Here's how the part is built. I have some questions about the finished solid (model axes, mm). A direction names the side the tool comes from. Coordinates: 2 decimals unless noted, no trailing zeros. Write each loop counter-clockwise with the first axis right and the second up, starting at its lowest first coordinate (ties: lowest second). Pieces come first, ordered by that corner, then holes.
Item 1: If we section it at D-D (z = 6.25): Please give me the cut outline in (x, y), then the cut area to 3 significant figures.
Item 2: We'd pull the mould along X, two halves only. Please class faces 3 (the face through (5, 2, 4)), 4 (the face through (-35, 2, 0)), 5 (the face through (35, 2, 0)), 6 (the face through (0, 2, 10)): +X half, -X half, draft (parallel to the pull), parting line (faces both ways), or undercut.
Item 3: If we section it at B-B (z = -3): Please give me the cut outline in (x, y), then the cut area to 3 significant figures.
Item 4: If we section it at A-A (x = -28.55): Please give me the cut outline in (y, z), then the cut area to 3 significant figures.
Item 5: For faces 1 (the face through (-5, 2, 4)), 2 (the face through (0, 2, -10)), which set-ups out of +Z, -Z, +X, -X, +Y, -Y let a thin tool reach every point of the face, with its end or its side?
Item 6: If we section it at C-C (y = 0.7): Please give me the cut outline in (x, z), then the cut area to 3 significant figures.
Item 7: If I drill on line 1 (X direction, y = 2, z = 1.5); line 2 (X direction, y = 3.05, z = -3); line 3 (Z direction, x = -30.5, y = 3.9), over which ranges is the centre line in solid material (lowest first)?
from build123d import *

# Parameters (mm, degrees)
SKETCH_1_W      = 70
SKETCH_1_H      = 20
SKETCH_1_R      = 3
SKETCH_1_W_2    = 2
SKETCH_1_H_2    = 7
EXTRUDE_1_DEPTH = 5


with BuildPart() as part:
    # 草图1 → 凸台-拉伸1 (new body)
    with BuildSketch(Plane(origin=(0, 0, 0), x_dir=(1, 0, 0), z_dir=(0, 1, 0))):
        Rectangle(SKETCH_1_W, SKETCH_1_H)
        with Locations(Location((-28.55, 3, 0), (0, 0, 270))):
            Circle(SKETCH_1_R, mode=Mode.SUBTRACT)
        with Locations(Location((28.55, 3, 0), (0, 0, 270))):
            Circle(SKETCH_1_R, mode=Mode.SUBTRACT)
        with Locations((-6, -3.5)):
            Rectangle(SKETCH_1_W_2, SKETCH_1_H_2, mode=Mode.SUBTRACT)
        with Locations((6, -3.5)):
            Rectangle(SKETCH_1_W_2, SKETCH_1_H_2, mode=Mode.SUBTRACT)
    extrude(amount=EXTRUDE_1_DEPTH)


solid = part.part
Answer list:
1. outline: (-35, 0) - (-7, 0) - (-7, 5) - (-35, 5) - close; (-5, 0) - (5, 0) - (5, 5) - (-5, 5) - close; (7, 0) - (35, 0) - (35, 5) - (7, 5) - close
1. area: 330 mm2
2. face 3: undercut
2. face 4: -X half
2. face 5: +X half
2. face 6: draft
3. outline: (-35, 0) - (-31.55, 0) - (-31.55, 5) - (-35, 5) - close; (-25.55, 0) - (25.55, 0) - (25.55, 5) - (-25.55, 5) - close; (31.55, 0) - (35, 0) - (35, 5) - (31.55, 5) - close
3. area: 290 mm2
4. outline: (0, -10) - (5, -10) - (5, -6) - (0, -6) - close; (0, 0) - (5, 0) - (5, 10) - (0, 10) - close
4. area: 70.0 mm2
5. face 1: +Y, -Y
5. face 2: -Z, +X, -X, +Y, -Y
6. outline: (-35, -10) - (35, -10) - (35, 10) - (-35, 10) - close; hole circle Ø6 at (-28.55, -3); hole (-7, 0) - (-5, 0) - (-5, 7) - (-7, 7) - close; hole (5, 0) - (7, 0) - (7, 7) - (5, 7) - close; hole circle Ø6 at (28.55, -3)
6. area: 1,320 mm2
7. line 1: x = -35 to -7, -5 to 5, 7 to 35
7. line 2: x = -35 to -31.55, -25.55 to 25.55, 31.55 to 35
7. line 3: z = -10 to -5.28, -0.72 to 10
